The drawing under review shows one solid part. Ordinate dimensions are in mm from its lowest x, y, z. Coordinates: 2 decimals unless noted, no trailing zeros. Write each loop counter-clockwise with the first axis right and the second up, starting at its lowest first coordinate (ties: lowest second). Pieces come first, ordered by that corner, then holes.
1) For line 1 (X direction, y = 93, z = 2.25); line 2 (X direction, y = 48.5, z = 6.25); line 3 (Y direction, x = 47, z = 5.75) (3 decimals), list the stretches that pass through material, from the lowest coordinate up.
2) Add section B-B, the plane x = 30.5. State the section outline as (y, z) points (3 decimals), then the cut area to 3 significant figures.
3) Add section C-C, the plane y = 119.5. State the section outline as (x, z) points.
4) Add section A-A, the plane z = 1.25. State the section outline as (x, y) points (3 decimals).
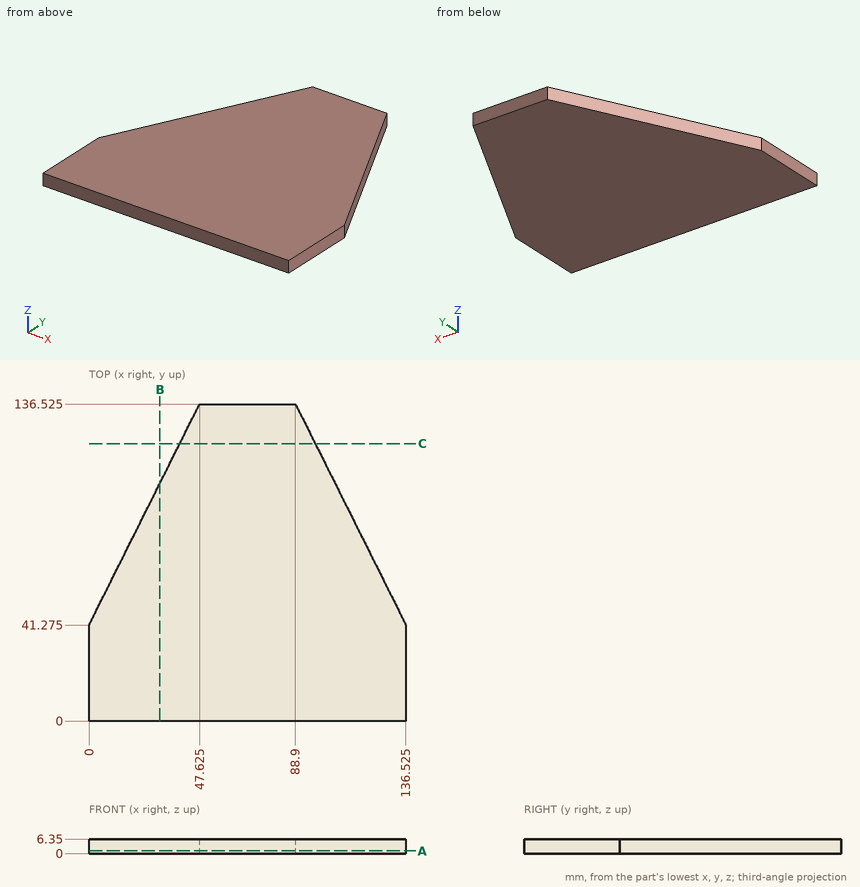
Geometry results:
1. line 1: x = 25.86 to 110.66
1. line 2: x = 3.61 to 132.91
1. line 3: y = 0 to 135.275
2. outline: (0, 0) - (102.275, 0) - (102.275, 6.35) - (0, 6.35) - close
2. area: 649 mm2
3. outline: (39.11, 0) - (97.41, 0) - (97.41, 6.35) - (39.11, 6.35) - close
4. outline: (0, 0) - (136.525, 0) - (136.525, 41.275) - (88.9, 136.525) - (47.625, 136.525) - (0, 41.275) - close
